The listing builds one solid part. Answer for the finished solid, in the listing's coordinates (mm). A direction names the side the tool comes from. Round coordinates to 2 decimals unless told otherwise and drop trailing zeros. Order: outer loops, then holes, each group sorted by start corner. A loop starts at its lowest first (then second) coordinate and runs counter-clockwise, first axis right, second up. Notation, with made-up numbers: (11, 34) - (41, 34) arc R27 cw to (41, 55) - close; hole circle Ø11 at (33.5, 74). An arc over 180 degrees is marked (long way). One line per item, written item: value. Start each with the question number.
1. Section D-D, the plane y = -20 is taken. Give the vertices of the cut face in (x, z), then the cut area to 3 significant figures.
2. Section C-C, the plane z = -9.5 is taken. Give the vertices of the cut face in (x, y), then the cut area to 3 significant figures.
3. Section A-A, the plane x = 0 is taken. Give the vertices of the cut face in (y, z).
4. Flat-ended cylindrical pins translate along their axes: P1, Ø12, axis at x = 17.5, z = -9.5, coming from the -Y side; P2, Ø6, axis at x = -2.5, z = -55, coming from the +Y side; P3, Ø1.5, axis at x = -5.5, z = -52, coming from the -Y side; P4, Ø8, axis at x = 0, y = 30, coming from the +Z side. Find the tip coordinate at first contact, or state that the pin passes through.
5. A tool of negligible diameter and unlimited length cuts with its end or side. For faces 5 (the flat face through (0, -11, -65)), 6 (the cylindrical face through (-23.846, 7.509, -44.72)), from which of +Z, -Z, +X, -X, +Y, -Y can it reach the whole face along a straight path? Write none if from no direction.
6. Section B-B, the plane y = 0 is taken. Give the vertices of the cut face in (x, z).
7. Straight lines are drawn through the part: line 1 (Y direction, x = 0, z = -19); line 2 (Z direction, x = -10.5, y = 33.5); line 3 (X direction, y = -2.5, z = -36.5). For each, find the intervals that lie inside material, in ascending order.
8. For a pull along X with two mould halves and no side action, classify faces 1 (the cylindrical face through (-2.17, -9.76, -32.04)), 2 (the cylindrical face through (-8.67, -39.05, -12.32)), 3 (the cylindrical face through (-0.46, 33.47, -12.32)), 4 (the flat face through (8, -8, 0)) as released by +X, released by -X, zero draft, split by the parting line, or undercut.
from build123d import *

# Parameters (mm, degrees)
SKETCH2_R           = 40
BOSS_EXTRUDE1_DEPTH = 25
SKETCH3_R           = 25
BOSS_EXTRUDE2_DEPTH = 40
SKETCH4_R           = 10
CUT_EXTRUDE1_DEPTH  = 87.168439698
SKETCH5_R           = 3.5
CUT_EXTRUDE2_DEPTH  = 87.168439698


with BuildPart() as part:
    # Sketch2 → Boss-Extrude1 (new body)
    with BuildSketch(Plane.XY):
        Circle(SKETCH2_R)
    extrude(amount=-BOSS_EXTRUDE1_DEPTH)

    # Sketch3 → Boss-Extrude2 (add)
    with BuildSketch(Plane(origin=(0, 0, -25), x_dir=(-1, 0, 0), z_dir=(0, 0, -1))):
        Circle(SKETCH3_R)
    extrude(amount=BOSS_EXTRUDE2_DEPTH)

    # Sketch4 → Cut-Extrude1 (cut, through all)
    with BuildSketch(Plane.XY):
        Circle(SKETCH4_R)
    extrude(amount=-CUT_EXTRUDE1_DEPTH, mode=Mode.SUBTRACT)

    # Sketch5 → Cut-Extrude2 (cut, through all)
    with BuildSketch(Plane.XY):
        with Locations((0, 30)):
            Circle(SKETCH5_R)
    extrude(amount=-CUT_EXTRUDE2_DEPTH, mode=Mode.SUBTRACT)


solid = part.part
Answer list:
1. outline: (-34.64, -25) - (-15, -25) - (-15, -65) - (15, -65) - (15, -25) - (34.64, -25) - (34.64, 0) - (-34.64, 0) - close
1. area: 2,930 mm²
2. outline: circle Ø80 at (0, 0); hole circle Ø20 at (0, 0); hole circle Ø7 at (0, 30)
2. area: 4,670 mm²
3. outline: (-40, -25) - (-25, -25) - (-25, -65) - (-10, -65) - (-10, 0) - (-40, 0) - close; (10, -65) - (25, -65) - (25, -25) - (26.5, -25) - (26.5, 0) - (10, 0) - close; (33.5, -25) - (40, -25) - (40, 0) - (33.5, 0) - close
4. P1: stops at y = -38.31
4. P2: stops at y = 25
4. P3: stops at y = -24.54
4. P4: stops at z = 0
5. face 5: -Z, +X, -X, +Y, -Y
5. face 6: -Z
6. outline: (-40, -25) - (-25, -25) - (-25, -65) - (-10, -65) - (-10, 0) - (-40, 0) - close; (10, -65) - (25, -65) - (25, -25) - (40, -25) - (40, 0) - (10, 0) - close
7. line 1: y = -40 to -10, 10 to 26.5, 33.5 to 40
7. line 2: z = -25 to 0
7. line 3: x = -24.87 to -9.68, 9.68 to 24.87
8. face 1: undercut
8. face 2: split by the parting line
8. face 3: undercut
8. face 4: zero draft
